Could you check a few things on this drawing? It's one solid part, dimensions in mm from its lowest x, y, z. Round coordinates to 2 decimals unless told otherwise and drop trailing zeros. Put each result on its own line as item: value.
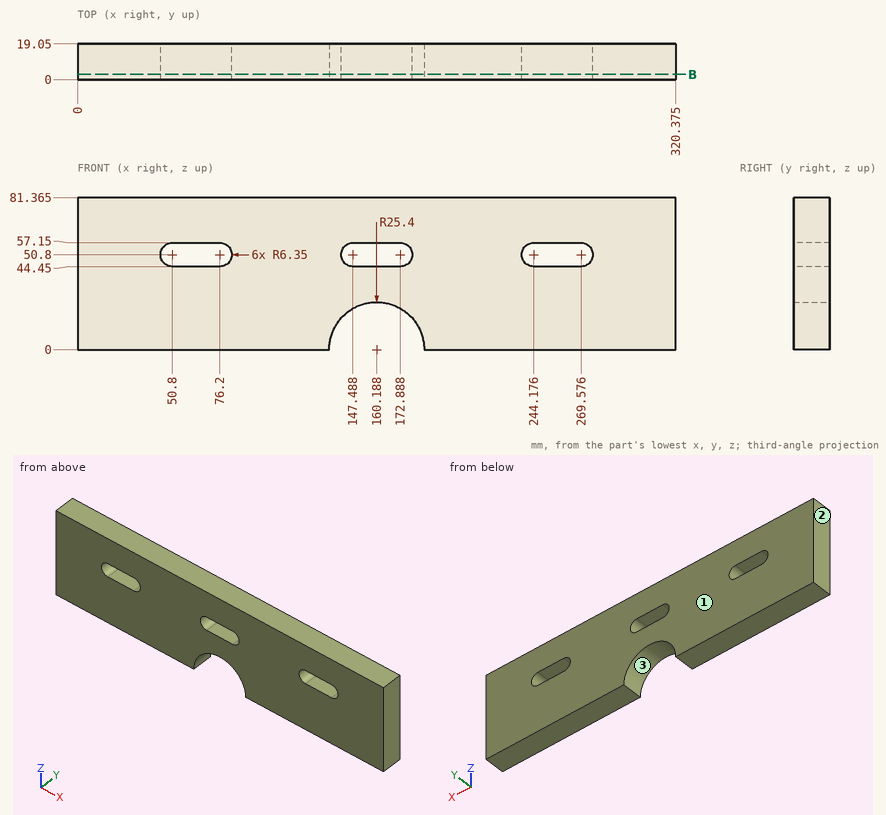
(1) I'm going to push a flat-ended pin straight in: pin 1 (5 mm diameter, centred on x = 164, y = 11, fed in from -Z). Where does the tip first touch, or does it pass through?
Values found:
pin 1: stops at z = 24.6
(2) Please list where these lines run through material, in increasing order: probe 1 along X at (y, z) = (12.75, 51.5) (1 decimal); probe 2 along X at (y, z) = (2.25, 53.5) (1 decimal); probe 3 along X at (y, z) = (11.25, 12) (1 decimal). Write a range as from..to.
Values found:
probe 1: x = 0..44.5, 82.5..141.2, 179.2..237.9, 275.9..320.4
probe 2: x = 0..45.1, 81.9..141.7, 178.6..238.4, 275.3..320.4
probe 3: x = 0..137.8, 182.6..320.4
(3) Imagine slicing it at B-B, the plane y = 2.75. Give the number of separate pieces and of enclosed holes in the cut face, then the cut area to 3 significant figures.
Values found:
separate pieces: 1
enclosed holes: 3
area: 23,700 mm^2
(4) If we mould it in two halves opening along X, with no side actions, what happens to the marked faces 1, 2 and 3? For each: pulls with the +X half, pulls with the -X half, needs draft (parallel to the pull), parting line crosses it, or undercut.
Values found:
face 1: needs draft
face 2: pulls with the -X half
face 3: undercut
